```python
from build123d import *

# Parameters (mm, degrees)
ESBO_O2_W                  = 3.3
ESBO_O2_H                  = 6.5
CORTE_EXTRUS_O1_DEPTH      = 13
CORTE_EXTRUS_O2_START      = -30
ESBO_O2_2_W                = 3.3
ESBO_O2_2_H                = 6.5
CORTE_EXTRUS_O2_DEPTH      = 13
CORTE_EXTRUS_O4_START      = 15
ESBO_O3_R                  = 1.65
CORTE_EXTRUS_O4_DEPTH      = 37.780782806
ESBO_O4_W                  = 59.68713318
ESBO_O4_H                  = 37
ESBO_O4_W_2                = 39.68713318
ESBO_O4_H_2                = 17
CORTE_EXTRUS_O_FINA1_DEPTH = 33


with BuildPart() as part:
    # Esboço1 → Revolução1 (revolve)
    with BuildSketch(Plane.XY):
        Polygon((4.5, 30), (15, 30), (15, 0), (3.25, 0), (3.25, 15), (4.5, 15), align=None)
    revolve(axis=Axis((0, 0, 0), (0, 1, 0)))

    # Esboço2 → Corte-extrusão1 (cut)
    with BuildSketch(Plane.XZ):
        with Locations((8.430782806, 0)):
            Rectangle(ESBO_O2_W, ESBO_O2_H)
        with Locations((-8.430782806, 0)):
            Rectangle(ESBO_O2_W, ESBO_O2_H)
    extrude(amount=-CORTE_EXTRUS_O1_DEPTH, mode=Mode.SUBTRACT)

    # Esboço2<2> → Corte-extrusão2 (cut)
    with BuildSketch(Plane.XZ.offset(CORTE_EXTRUS_O2_START)):
        with Locations((8.430782806, 0)):
            Rectangle(ESBO_O2_2_W, ESBO_O2_2_H)
        with Locations((-8.430782806, 0)):
            Rectangle(ESBO_O2_2_W, ESBO_O2_2_H)
    extrude(amount=CORTE_EXTRUS_O2_DEPTH, mode=Mode.SUBTRACT)

    # Esboço3 → Corte-extrusão4 (cut, through all)
    with BuildSketch(Plane(origin=(6.780782806, 0, 0), x_dir=(0, 0, -1), z_dir=(1, 0, 0)).offset(CORTE_EXTRUS_O4_START)):
        with Locations((0, 23.5)):
            Circle(ESBO_O3_R)
        with Locations((0, 6.5)):
            Circle(ESBO_O3_R)
    extrude(amount=-CORTE_EXTRUS_O4_DEPTH, mode=Mode.SUBTRACT)

    # Esboço4 → Corte-Extrusão-Fina1 (cut)
    with BuildSketch(Plane.XZ):
        Rectangle(ESBO_O4_W, ESBO_O4_H)
        Rectangle(ESBO_O4_W_2, ESBO_O4_H_2, mode=Mode.SUBTRACT)
    extrude(amount=-CORTE_EXTRUS_O_FINA1_DEPTH, mode=Mode.SUBTRACT)


solid = part.part
```
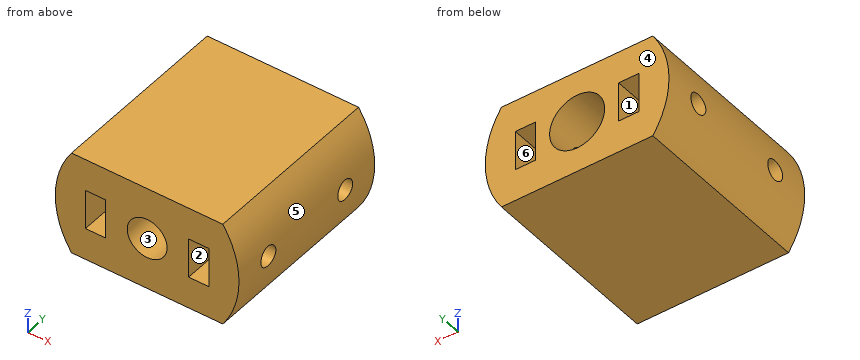
Check sheet for the modelled part. Datum: model origin and axes. Units: mm. Face numbers are marked on the shaded views. A direction names the side the tool comes from. Give positions to 0.01 mm unless a question says otherwise; leave off trailing zeros. Loops run counter-clockwise (first coordinate to the right, second up) from the corner with the lowest first, then second, coordinate; pieces in that order, holes last. Notation, with made-up numbers: (28.25, 8) - (57.25, 8) arc R26 cw to (57.25, 40) - close; hole circle Ø5 at (13, 78.5). An arc over 180 degrees is marked (long way). One line per question, with ' | ' between items. Start each with the question number.
1. Cross-section at D-D, the plane x = -5.5. Enter the section's corners in (y, z).
2. Material ranges on line 1 along X through (y, z) = (4, 0); line 2 along X through (y, z) = (27, 0); line 3 along Y through (x, z) = (-5.8, 0), recorded low to high. Write a range as [from, to].
3. Cross-section at A-A, the plane x = 0. Enter the section's corners in (y, z), plus the area to 4 significant figures.
4. Set-up check for the marked faces 1, 2 and 3: record each of +Z, -Z, +X, -X, +Y, -Y from which the full face is reachable in a straight line by a thin tool's end or side.
5. Gauge pin test, flat ends, axial feed: pin 1 Ø3 at (y, z) = (25, -2.5) entering from +X; pin 2 Ø2.5 at (y, z) = (23.5, 0) entering from +X; pin 3 Ø1.5 at (y, z) = (10, 2.5) entering from +X; pin 4 Ø1.5 at (y, z) = (26, 4) entering from -X. Record the tip position at first contact, or that the pin passes through.
6. Cross-section at C-C, the plane y = 22.5. Enter the section's corners in (x, z).
7. Cross-section at B-B, the plane y = 3.5. Enter the section's corners in (x, z).
8. Draft check along Z on the marked faces 4, 5 and 6. Enter one of: released by +Z, released by -Z, zero draft, split by the parting line, or undercut.
Check result:
1) outline: (0, -8.5) - (30, -8.5) - (30, 8.5) - (0, 8.5) - close; hole circle Ø3.3 at (6.5, 0); hole circle Ø3.3 at (23.5, 0)
2) line 1: x = [-15, -10.08], [-6.78, -3.25], [3.25, 6.78], [10.08, 15] | line 2: x = [-15, -10.08], [-6.78, -4.5], [4.5, 6.78], [10.08, 15] | line 3: y = [0, 4.85], [8.15, 21.85], [25.15, 30]
3) outline: (0, -8.5) - (30, -8.5) - (30, -4.5) - (15, -4.5) - (15, -3.25) - (0, -3.25) - close; (0, 3.25) - (15, 3.25) - (15, 4.5) - (30, 4.5) - (30, 8.5) - (0, 8.5) - close | area: 277.5 mm2
4) face 1: +Y | face 2: -Y | face 3: +Y, -Y
5) pin 1: stops at x = 14.97 | pin 2: passes through | pin 3: stops at x = 14.9 | pin 4: stops at x = -14.64
6) outline: (-14.94, -1.31) arc R15 ccw to (-12.36, -8.5) - (12.36, -8.5) arc R15 ccw to (14.94, -1.31) - (10.08, -1.31) - (10.08, -3.25) - (6.78, -3.25) - (6.78, -1.31) - (4.3, -1.31) arc R4.5 cw to (-4.3, -1.31) - (-6.78, -1.31) - (-6.78, -3.25) - (-10.08, -3.25) - (-10.08, -1.31) - close; (-14.94, 1.31) - (-10.08, 1.31) - (-10.08, 3.25) - (-6.78, 3.25) - (-6.78, 1.31) - (-4.3, 1.31) arc R4.5 cw to (4.3, 1.31) - (6.78, 1.31) - (6.78, 3.25) - (10.08, 3.25) - (10.08, 1.31) - (14.94, 1.31) arc R15 ccw to (12.36, 8.5) - (-12.36, 8.5) arc R15 ccw to start
7) outline: (-12.36, -8.5) - (12.36, -8.5) arc R15 ccw to (12.36, 8.5) - (-12.36, 8.5) arc R15 ccw to start; hole (-10.08, -3.25) - (-6.78, -3.25) - (-6.78, 3.25) - (-10.08, 3.25) - close; hole circle Ø6.5 at (0, 0); hole (6.78, -3.25) - (10.08, -3.25) - (10.08, 3.25) - (6.78, 3.25) - close
8) face 4: zero draft | face 5: split by the parting line | face 6: undercut
